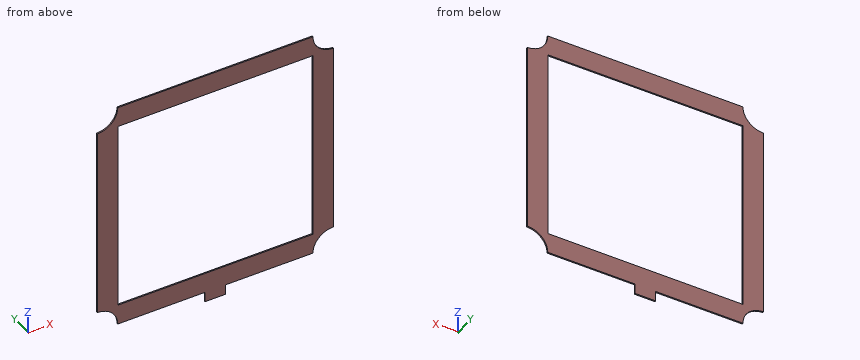
from build123d import *

# Parameters (mm, degrees)
SKETCH1_W           = 120.65
SKETCH1_H           = 120.65
BOSS_EXTRUDE1_DEPTH = 0.8
SKETCH2_W           = 12.7
SKETCH2_H           = 6.35
BOSS_EXTRUDE2_DEPTH = 0.8


with BuildPart() as part:
    # Sketch1 → Boss-Extrude1 (new body)
    with BuildSketch(Plane(origin=(0, 0, 0), x_dir=(1, 0, 0), z_dir=(0, 1, 0))):
        with BuildLine():
            Line((69.867533733, 87.286057649), (-50.782466267, 87.286057649))
            ThreePointArc((-50.782466267, 87.286057649), (-54.502210146, 78.305801528), (-63.482466267, 74.586057649))
            Line((-63.482466267, 74.586057649), (-63.482466267, -46.063942351))
            ThreePointArc((-63.482466267, -46.063942351), (-54.502210146, -49.78368623), (-50.782466267, -58.763942351))
            Line((-50.782466267, -58.763942351), (69.867533733, -58.763942351))
            ThreePointArc((69.867533733, -58.763942351), (73.587277612, -49.78368623), (82.567533733, -46.063942351))
            Line((82.567533733, -46.063942351), (82.567533733, 74.586057649))
            ThreePointArc((82.567533733, 74.586057649), (73.587277612, 78.305801528), (69.867533733, 87.286057649))
        make_face()
        with Locations((9.542533733, 14.261057649)):
            Rectangle(SKETCH1_W, SKETCH1_H, mode=Mode.SUBTRACT)
    extrude(amount=BOSS_EXTRUDE1_DEPTH)

    # Sketch2 → Boss-Extrude2 (add)
    with BuildSketch(Plane(origin=(0, 0.8, 0), x_dir=(1, 0, 0), z_dir=(0, 1, 0))):
        with Locations((9.542533733, 90.461057649)):
            Rectangle(SKETCH2_W, SKETCH2_H)
    extrude(amount=-BOSS_EXTRUDE2_DEPTH)


solid = part.part
The listing builds one solid part. Answer for the finished solid, in the listing's coordinates (mm). Round coordinates to 2 decimals unless told otherwise and drop trailing zeros. Order: outer loops, then holes, each group sorted by start corner. A loop starts at its lowest first (then second) coordinate and runs counter-clockwise, first axis right, second up. Notation, with made-up numbers: (0.5, -22.75) -> (8.5, -22.75) arc R21 cw to (8.5, -9.75) -> close; hole circle Ø7 at (22.25, 29). An arc over 180 degrees is marked (long way). Put each result on its own line as item: value.
Q1. Consider line 1 along X through (y, z) = (0.5, -21); line 2 along Z through (x, y) = (4.5, 0.1); line 3 along Z through (x, y) = (-44, 0.7). Determine where each line is inside the solid, lowest interval first.
Results list:
line 1: -63.48 to -50.78, 69.87 to 82.57
line 2: -93.64 to -74.59, 46.06 to 58.76
line 3: -87.29 to -74.59, 46.06 to 58.76
Q2. Section B-B, the plane z = -70.5 is taken. Write down the section's boundary in (x, y).
Results list:
outline: (-63.48, 0) -> (-50.78, 0) -> (-50.78, 0.8) -> (-63.48, 0.8) -> close; (69.87, 0) -> (82.57, 0) -> (82.57, 0.8) -> (69.87, 0.8) -> close
Q3. Section C-C, the plane y = 0.55 is taken. Write down the section's boundary in (x, z).
Results list:
outline: (-63.48, -74.59) arc R12.7 cw to (-50.78, -87.29) -> (3.19, -87.29) -> (3.19, -93.64) -> (15.89, -93.64) -> (15.89, -87.29) -> (69.87, -87.29) arc R12.7 cw to (82.57, -74.59) -> (82.57, 46.06) arc R12.7 cw to (69.87, 58.76) -> (-50.78, 58.76) arc R12.7 cw to (-63.48, 46.06) -> close; hole (-50.78, -74.59) -> (69.87, -74.59) -> (69.87, 46.06) -> (-50.78, 46.06) -> close
Q4. This flat-tipped pin is pushed along its axis until it touches: P1, Ø8, axis at x = 41, z = -75, coming from the -Y side. Where does it stop, or does it pass through?
Results list:
P1: y = 0
Q5. Section A-A, the plane x = -26.5 is taken. Write down the section's boundary in (y, z).
Results list:
outline: (0, -87.29) -> (0.8, -87.29) -> (0.8, -74.59) -> (0, -74.59) -> close; (0, 46.06) -> (0.8, 46.06) -> (0.8, 58.76) -> (0, 58.76) -> close
Q6. Section D-D, the plane x = -53 is taken. Write down the section's boundary in (y, z).
Results list:
outline: (0, -80.12) -> (0.8, -80.12) -> (0.8, 51.59) -> (0, 51.59) -> close
